```python
from build123d import *

# Parameters (mm, degrees)
F0_R     = 1.5
F1_DEPTH = 50
F2_R     = 1
F3_DEPTH = 50.001
F4_R     = 1.5
F4_R_2   = 1
F5_R     = 3
F5_R_2   = 1.5
F6_DEPTH = 1


with BuildPart() as f1:
    # F0 (on Front) → F1 (new body)
    with BuildSketch(Plane.XZ):
        Circle(F0_R)
    extrude(amount=F1_DEPTH)

    # F2 (on face) → F3 (cut, through all)
    with BuildSketch(Plane.XZ.offset(50)):
        Circle(F2_R)
    extrude(amount=-F3_DEPTH, mode=Mode.SUBTRACT)

    # F4 (on face) + F5 (on face) → F6 (join)
    with BuildSketch(Plane.XZ.offset(50)):
        Circle(F4_R)
        Circle(F4_R_2, mode=Mode.SUBTRACT)
    with BuildSketch(Plane.XZ.offset(50)):
        Circle(F5_R)
        Circle(F5_R_2, mode=Mode.SUBTRACT)
    extrude(amount=F6_DEPTH)


solid = f1.part
```
Geometry: final body of the model. Coordinates: model frame, mm. Give positions to 0.01 mm unless a question says otherwise; leave off trailing zeros. Order: outer loops, then holes, each group sorted by start corner. A loop starts at its lowest first (then second) coordinate and runs counter-clockwise, first axis right, second up. Notation, with made-up numbers: M -24.5,75 L -19.5,75 A18 ccw -19.5,107 Z; hole C -14.75,-28.75 d5. An arc over 180 degrees is marked long. Answer as CSV lines item,"result". Start each with the question number.
1) Line query: line 1 (X direction, y = -9, z = -0.05); line 2 (Z direction, x = 0, y = -50.8); line 3 (Z direction, x = 0.1, y = -12). Output: solid intervals per line, ascending. Write a range as from..to.
2) Cut plane A-A (x = 0). Output: boundary loops of the cut face in (y, z).
3) Cut plane C-C (y = -18.5). Output: boundary loops of the cut face in (x, z), then the cut area to 3 significant figures.
4) First-contact query: P1, Ø3, axis at y = -8, z = 0, coming from the +X side; P2, Ø3, axis at y = -12.5, z = -2, coming from the -X side. Flat tips, straight axial feed; report the tip coordinate or a pass-through.
5) Mould query, pull axis Y, two halves, no side actions, for faces 1 (the flat face through (1.3, -50, -1.3)), 2 (the cylindrical face through (-3, -50.5, 0.1)). Classes: +Y half, -Y half, draft (parallel to the pull), parting line (faces both ways), or undercut.
6) Cut plane D-D (z = -2.2). Output: boundary loops of the cut face in (x, y).
7) Cut plane B-B (z = 0). Output: boundary loops of the cut face in (x, y).
Findings below:
1,line 1,"x = -1.5..-1, 1..1.5"
1,line 2,"z = -3..-1, 1..3"
1,line 3,"z = -1.5..-0.99, 0.99..1.5"
2,outline,"M -51,-3 L -50,-3 L -50,-1.5 L 0,-1.5 L 0,-1 L -51,-1 Z; M -51,1 L 0,1 L 0,1.5 L -50,1.5 L -50,3 L -51,3 Z"
3,outline,"C 0,0 d3; hole C 0,0 d2"
3,area,"3.93 mm²"
4,P1,"stops at x = 1.5"
4,P2,"stops at x = -1.41"
5,face 1,"+Y half"
5,face 2,"draft"
6,outline,"M -2.04,-51 L 2.04,-51 L 2.04,-50 L -2.04,-50 Z"
7,outline,"M -3,-51 L -1,-51 L -1,0 L -1.5,0 L -1.5,-50 L -3,-50 Z; M 1,-51 L 3,-51 L 3,-50 L 1.5,-50 L 1.5,0 L 1,0 Z"
